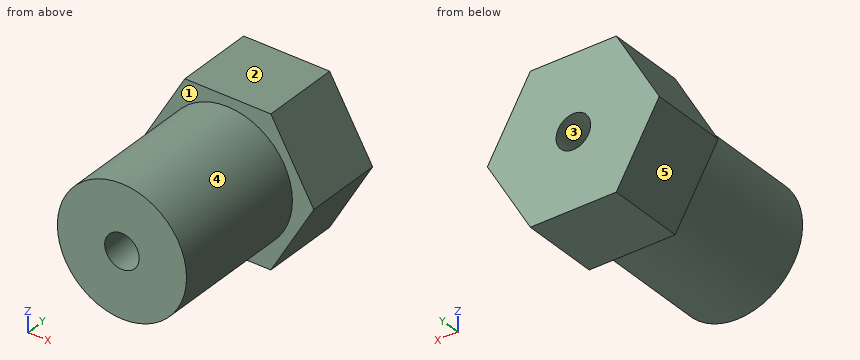
```python
from build123d import *

# Parameters (mm, degrees)
SKETCH1_R           = 5.2324
BOSS_EXTRUDE1_DEPTH = 11.43
BOSS_EXTRUDE2_DEPTH = 6.35
SKETCH3_R           = 1.397
CUT_EXTRUDE1_DEPTH  = 18.78


with BuildPart() as part:
    # Sketch1 → Boss-Extrude1 (new body)
    with BuildSketch(Plane(origin=(0, 0, 0), x_dir=(1, 0, 0), z_dir=(0, 1, 0))):
        Circle(SKETCH1_R)
    extrude(amount=BOSS_EXTRUDE1_DEPTH)

    # Sketch2 → Boss-Extrude2 (add)
    with BuildSketch(Plane(origin=(0, 11.43, 0), x_dir=(1, 0, 0), z_dir=(0, 1, 0))):
        Polygon((6.965730998, 0), (3.482865499, 6.0325), (-3.482865499, 6.0325), (-6.965730998, 0), (-3.482865499, -6.0325), (3.482865499, -6.0325), align=None)
    extrude(amount=BOSS_EXTRUDE2_DEPTH)

    # Sketch3 → Cut-Extrude1 (cut, through all)
    with BuildSketch(Plane(origin=(0, 17.78, 0), x_dir=(1, 0, 0), z_dir=(0, 1, 0))):
        Circle(SKETCH3_R)
    extrude(amount=-CUT_EXTRUDE1_DEPTH, mode=Mode.SUBTRACT)


solid = part.part
```
CAD build for the part. Positions are in the model's coordinates, mm. Face numbers are marked on the shaded views. A direction names the side the tool comes from. Coordinates: 2 decimals unless noted, no trailing zeros. Order: outer loops, then holes, each group sorted by start corner. A loop starts at its lowest first (then second) coordinate and runs counter-clockwise, first axis right, second up. Notation, with made-up numbers: (-34.75, 36) - (22.25, 36) arc R14 ccw to (22.25, 63) - close; hole circle Ø1 at (89, -24). An arc over 180 degrees is marked (long way). Answer in a Markdown table with one row per item.
1. Flat gauge pins, fed straight in: P1, Ø1.5, axis at y = 14, z = -4.5, coming from the -X side; P2, Ø8, axis at x = 3.5, y = 3, coming from the -Z side; P3, Ø1.5, axis at y = 14.5, z = 4.5, coming from the +X side. Where does each tip first touch, or does it go through?
Answer:
| item | result |
|---|---|
| P1 | x = -4.8 |
| P2 | z = -5.23 |
| P3 | x = 4.8 |
2. Slice it at B-B, the plane y = 14.5. List the corners of the cut face in (x, z), then the cut area to 3 significant figures.
Answer:
| item | result |
|---|---|
| outline | (-6.97, 0) - (-3.48, -6.03) - (3.48, -6.03) - (6.97, 0) - (3.48, 6.03) - (-3.48, 6.03) - close; hole circle Ø2.79 at (0, 0) |
| area | 120 mm² |
3. 3-axis set-ups, long thin cutter, end or side, ignore diameter. For the marked faces 4 and 5: which of +Z, -Z, +X, -X, +Y, -Y reach the whole face in a straight line?
Answer:
| item | result |
|---|---|
| face 4 | -Y |
| face 5 | -Z, -X, +Y, -Y |
4. Pull direction Z, two halves, no side cores. Call the marked faces 1, 2 and 3: +Z half, -Z half, draft (parallel to the pull), parting line (faces both ways), or undercut.
Answer:
| item | result |
|---|---|
| face 1 | draft |
| face 2 | +Z half |
| face 3 | undercut |
5. Slice it at C-C, the plane z = 2.75. List the corners of the cut face in (x, y).
Answer:
| item | result |
|---|---|
| outline | (-5.38, 11.43) - (-4.45, 11.43) - (-4.45, 0) - (4.45, 0) - (4.45, 11.43) - (5.38, 11.43) - (5.38, 17.78) - (-5.38, 17.78) - close |
6. Slice it at A-A, the plane x = 0. List the corners of the cut face in (y, z), then the cut area to 3 significant figures.
Answer:
| item | result |
|---|---|
| outline | (0, -5.23) - (11.43, -5.23) - (11.43, -6.03) - (17.78, -6.03) - (17.78, -1.4) - (0, -1.4) - close; (0, 1.4) - (17.78, 1.4) - (17.78, 6.03) - (11.43, 6.03) - (11.43, 5.23) - (0, 5.23) - close |
| area | 147 mm² |
7. Drill centre lines: L1, parallel to X at y = 4.25, z = 0; L2, parallel to Y at x = 5, z = -2. Where is each one in solid material? Low to high. Write a range as from..to.
Answer:
| item | result |
|---|---|
| L1 | -5.23..-1.4, 1.4..5.23 |
| L2 | 11.43..17.78 |
8. Slice it at D-D, the plane x = -4.5. List the corners of the cut face in (y, z), then the cut area to 3 significant figures.
Answer:
| item | result |
|---|---|
| outline | (0, -2.67) - (11.43, -2.67) - (11.43, -4.27) - (17.78, -4.27) - (17.78, 4.27) - (11.43, 4.27) - (11.43, 2.67) - (0, 2.67) - close |
| area | 115 mm² |
